Design review of the part built by this model. Coordinates are the model's own, in mm. Round coordinates to 2 decimals unless told otherwise and drop trailing zeros. Write each loop counter-clockwise with the first axis right and the second up, starting at its lowest first coordinate (ties: lowest second). Pieces come first, ordered by that corner, then holes. Notation, with made-up numbers: (83.5, 59) -> (88.5, 59) arc R10 ccw to (88.5, 68) -> close; hole circle Ø11 at (19.25, 10.5). An arc over 180 degrees is marked (long way). Write item = value, one per line. Start each with the question number.
Item 1: Add section C-C, the plane z = 0.3. State the section outline as (x, y) points.
Item 2: For pin 1 Ø0.6 at (y, z) = (16, 0.5) entering from +X, flat-tipped, find the tip position at first contact; note if it passes through.
Item 3: To check wall thickness, follow L1, parallel to Y at x = 12, z = 1.05; L2, parallel to Y at x = -5, z = 1.05; L3, parallel to X at y = 10.5, z = 1. State the ranges of each line that lie inside material, in increasing order.
Item 4: Add section D-D, the plane x = -1. State the section outline as (y, z) points.
Item 5: Add section A-A, the plane x = -7.5. State the section outline as (y, z) points.
Item 6: Add section B-B, the plane y = 7. State the section outline as (x, z) points.
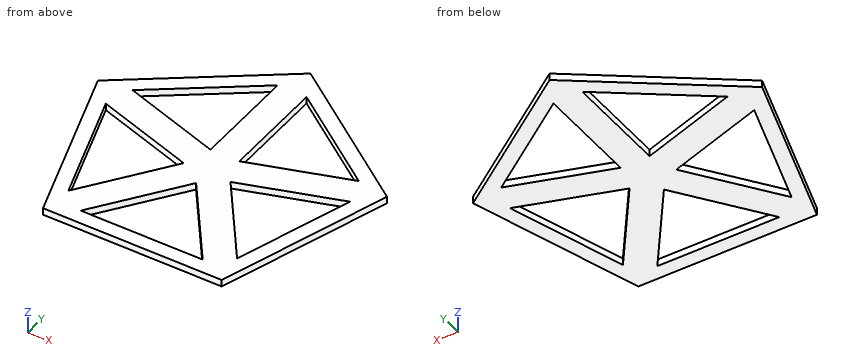
from build123d import *

# Parameters (mm, degrees)
BOSS_EXTRUDE1_DEPTH = 1.2


with BuildPart() as part:
    # Sketch1 → Boss-Extrude1 (new body)
    with BuildSketch(Plane.XY):
        Polygon((0, 26.286555606), (-25, 8.122992406), (-15.450849719, -21.266270209), (15.450849719, -21.266270209), (25, 8.122992406), align=None)
        Polygon((-21.10615871, 4.229151116), (-4.045084972, -1.31432778), (-14.589408427, -15.827343947), align=None, mode=Mode.SUBTRACT)
        Polygon((14.589408427, -15.827343947), (21.10615871, 4.229151116), (4.045084972, -1.31432778), align=None, mode=Mode.SUBTRACT)
        Polygon((-19.561073739, 8.984433698), (-2.5, 3.440954801), (-2.5, 21.380029342), align=None, mode=Mode.SUBTRACT)
        Polygon((2.5, 21.380029342), (2.5, 3.440954801), (19.561073739, 8.984433698), align=None, mode=Mode.SUBTRACT)
        Polygon((-10.544323455, -18.766270209), (0, -4.253254042), (10.544323455, -18.766270209), align=None, mode=Mode.SUBTRACT)
    extrude(amount=BOSS_EXTRUDE1_DEPTH)


solid = part.part
Result set:
q1.outline = (-25, 8.12) -> (-15.45, -21.27) -> (15.45, -21.27) -> (25, 8.12) -> (0, 26.29) -> close; hole (-21.11, 4.23) -> (-14.59, -15.83) -> (-4.05, -1.31) -> close; hole (-19.56, 8.98) -> (-2.5, 3.44) -> (-2.5, 21.38) -> close; hole (-10.54, -18.77) -> (10.54, -18.77) -> (0, -4.25) -> close; hole (2.5, 3.44) -> (19.56, 8.98) -> (2.5, 21.38) -> close; hole (4.05, -1.31) -> (14.59, -15.83) -> (21.11, 4.23) -> close
q2.pin_1 = 14.57
q3.L1 = -21.27 to -12.26, 1.27 to 6.53, 14.48 to 17.57
q3.L2 = -21.27 to -18.77, -11.14 to -2.63, -1 to 4.25, 19.56 to 22.65
q3.L3 = -21.73 to -17.48, -2.5 to 2.5, 17.48 to 21.73
q4.outline = (-21.27, 0) -> (-18.77, 0) -> (-18.77, 1.2) -> (-21.27, 1.2) -> close; (-5.63, 0) -> (25.56, 0) -> (25.56, 1.2) -> (-5.63, 1.2) -> close
q5.outline = (-21.27, 0) -> (-18.77, 0) -> (-18.77, 1.2) -> (-21.27, 1.2) -> close; (-14.58, 0) -> (-6.07, 0) -> (-6.07, 1.2) -> (-14.58, 1.2) -> close; (-0.19, 0) -> (5.07, 0) -> (5.07, 1.2) -> (-0.19, 1.2) -> close; (17.75, 0) -> (20.84, 0) -> (20.84, 1.2) -> (17.75, 1.2) -> close
q6.outline = (-24.64, 0) -> (-13.45, 0) -> (-13.45, 1.2) -> (-24.64, 1.2) -> close; (-2.5, 0) -> (2.5, 0) -> (2.5, 1.2) -> (-2.5, 1.2) -> close; (13.45, 0) -> (24.64, 0) -> (24.64, 1.2) -> (13.45, 1.2) -> close
